Can you work these out from the model? Positions are in its coordinate system, mm. A direction names the side the tool comes from. Round coordinates to 2 decimals unless told otherwise and drop trailing zeros. Write each loop counter-clockwise with the first axis right and the second up, starting at its lowest first coordinate (ties: lowest second). Pieces come first, ordered by that corner, then holes. Notation, with made-up numbers: M 79,13 L 116,13 A28 cw 116,34 Z; hole C 8,-3 d2. An arc over 180 degrees is marked long. Use one line per item in the form item = value. Start each with the question number.
```python
from build123d import *

# Parameters (mm, degrees)
ESQUISSE1_W             = 37
ESQUISSE1_H             = 42.25
ESQUISSE1_R             = 6
BOSS_EXTRU_1_DEPTH      = 12
ESQUISSE2_R             = 6
ESQUISSE2_R_2           = 1.5
ENL_V_MAT_EXTRU_1_DEPTH = 3
ESQUISSE3_W             = 37
ESQUISSE3_H             = 12
ESQUISSE3_W_2           = 15.75
ESQUISSE3_R             = 2.75
BOSS_EXTRU_2_DEPTH      = 3
ESQUISSE4_W             = 37
ESQUISSE4_H             = 45.25
ESQUISSE4_R             = 8
ENL_V_MAT_EXTRU_2_DEPTH = 4
ESQUISSE4_3_R           = 8
ESQUISSE4_3_R_2         = 6
ESQUISSE4_3_R_3         = 1.5
ENL_V_MAT_EXTRU_4_DEPTH = 7
CONG_2_R                = 5
CONG_3_R                = 5
ESQUISSE5_R             = 2
ENL_V_MAT_EXTRU_5_DEPTH = 43.650652105
BOSS_EXTRU_3_START      = 2
ESQUISSE2_2_R           = 1.5
BOSS_EXTRU_3_DEPTH      = 2
SYM_TRIE1_OUTLINE_W     = 37
SYM_TRIE1_OUTLINE_H     = 45.25
SYM_TRIE1_OUTLINE_R     = 8
SYM_TRIE1_OUTLINE_R_2   = 2
SYM_TRIE1_OUTLINE_R_3   = 1.5
SYM_TRIE1_DEPTH         = 8
SYM_TRIE1_2_OUTLINE_W   = 15.75
SYM_TRIE1_2_OUTLINE_H   = 3
SYM_TRIE1_2_OUTLINE_R   = 8
SYM_TRIE1_2_OUTLINE_R_2 = 1.5
SYM_TRIE1_2_DEPTH       = 4.7499999
SYM_TRIE1_START         = 10.2500001
SYM_TRIE1_3_OUTLINE_W   = 15.75
SYM_TRIE1_3_OUTLINE_H   = 3
SYM_TRIE1_3_OUTLINE_R   = 1.5
SYM_TRIE1_3_DEPTH       = 1.7499999
SYM_TRIE1_START_2       = 1.13256
SYM_TRIE1_4_OUTLINE_R   = 8
SYM_TRIE1_4_OUTLINE_R_2 = 1.5
SYM_TRIE1_4_DEPTH       = 3.86744
SYM_TRIE1_START_3       = 8
SYM_TRIE1_5_OUTLINE_R   = 1.5
SYM_TRIE1_5_DEPTH       = 2.73256
SYM_TRIE1_START_4       = -24.125
SYM_TRIE1_6_DEPTH       = 3
ESQUISSE6_W             = 14
ESQUISSE6_H             = 45.25
ENL_V_MAT_EXTRU_6_DEPTH = 60.670580063


with BuildPart() as part:
    # Esquisse1 → Boss.-Extru.1 (new body)
    # profile 1 of 2: a face of its own
    with BuildSketch(Plane.XY):
        Rectangle(ESQUISSE1_W, ESQUISSE1_H)
        with Locations((3.4, 9.125)):
            Circle(ESQUISSE1_R, mode=Mode.SUBTRACT)
    # profile 2 of 2: a face of its own
    with BuildSketch(Plane.XY):
        with Locations((3.4, 9.125)):
            Circle(ESQUISSE1_R)
    extrude(amount=BOSS_EXTRU_1_DEPTH)

    # Esquisse2 → Enlèv. mat.-Extru.1 (cut)
    with BuildSketch(Plane.XY.offset(12)):
        with Locations((3.4, 9.125)):
            Circle(ESQUISSE2_R)
        with Locations((3.4, 9.125)):
            Circle(ESQUISSE2_R_2, mode=Mode.SUBTRACT)
    extrude(amount=-ENL_V_MAT_EXTRU_1_DEPTH, mode=Mode.SUBTRACT)

    # Esquisse3 → Boss.-Extru.2 (add)
    # profile 1 of 2: a face of its own
    with BuildSketch(Plane.XZ.offset(21.125)):
        with Locations((0, 6)):
            Rectangle(ESQUISSE3_W, ESQUISSE3_H)
    # profile 2 of 2: a face of its own
    with BuildSketch(Plane.XZ.offset(21.125)):
        with Locations((-26.375, 6)):
            Rectangle(ESQUISSE3_W_2, ESQUISSE3_H)
        with Locations((-29, 7.5)):
            Circle(ESQUISSE3_R, mode=Mode.SUBTRACT)
    extrude(amount=BOSS_EXTRU_2_DEPTH)

    # Esquisse4 → Enlèv. mat.-Extru.2 (cut)
    with BuildSketch(Plane.XY.offset(12)):
        with Locations((0, -1.5)):
            Rectangle(ESQUISSE4_W, ESQUISSE4_H)
        with Locations((3.4, 9.125)):
            Circle(ESQUISSE4_R, mode=Mode.SUBTRACT)
    extrude(amount=-ENL_V_MAT_EXTRU_2_DEPTH, mode=Mode.SUBTRACT)

    # Esquisse4<3> → Enlèv. mat.-Extru.4 (cut)
    # profile 1 of 2: a face of its own
    with BuildSketch(Plane.XY.offset(12)):
        with Locations((3.4, 9.125)):
            Circle(ESQUISSE4_3_R)
        with Locations((3.4, 9.125)):
            Circle(ESQUISSE4_3_R_2, mode=Mode.SUBTRACT)
    # profile 2 of 2: a face of its own
    with BuildSketch(Plane.XY.offset(12)):
        with Locations((3.4, 9.125)):
            Circle(ESQUISSE4_3_R_2)
        with Locations((3.4, 9.125)):
            Circle(ESQUISSE4_3_R_3, mode=Mode.SUBTRACT)
    extrude(amount=-ENL_V_MAT_EXTRU_4_DEPTH, mode=Mode.SUBTRACT)

    # Congé2
    # the kernel refuses this fillet: 5 mm, written as the material it adds along each edge
    with BuildSketch(Plane(origin=(-18.5, -24.125, 8), x_dir=(1.5667467323505199e-12, 0, 1.0), z_dir=(0, 1, 0))) as cong_2_piece_1:
        with BuildLine():
            CenterArc((5, 4.898979486), CONG_2_R, 180, 78.463040967)
            Line((0, 4.898979486), (0, 0))
            Line((0, 0), (4, 0))
        make_face()
    extrude(amount=3)

    # Congé3
    cong_3_edges = [part.edges().sort_by_distance(p)[0] for p in [
        (-18.5, -22.625, 12),
    ]]
    fillet(cong_3_edges, radius=CONG_3_R)

    # Esquisse5 → Enlèv. mat.-Extru.5 (cut, through all)
    with BuildSketch(Plane.XY.offset(8)):
        with Locations((-12, 16.625)):
            Circle(ESQUISSE5_R)
        with Locations((-12, 4.625)):
            Circle(ESQUISSE5_R)
        with Locations((15.5, 10.625)):
            Circle(ESQUISSE5_R)
    extrude(amount=-ENL_V_MAT_EXTRU_5_DEPTH, mode=Mode.SUBTRACT)

    # Esquisse2<2> → Boss.-Extru.3 (add)
    with BuildSketch(Plane.XY.offset(12).offset(BOSS_EXTRU_3_START)):
        with Locations((3.4, 9.125)):
            Circle(ESQUISSE2_2_R)
    extrude(amount=-BOSS_EXTRU_3_DEPTH)

    # Symétrie1: read off the stored shape, not the designer's step
    # Symétrie1 outline → Symétrie1 (add)
    # profile 1 of 2: a face of its own
    with BuildSketch(Plane.XY):
        with Locations((37, -1.5)):
            Rectangle(SYM_TRIE1_OUTLINE_W, SYM_TRIE1_OUTLINE_H)
        with Locations((33.6, 9.125)):
            Circle(SYM_TRIE1_OUTLINE_R, mode=Mode.SUBTRACT)
        with Locations((21.5, 10.625)):
            Circle(SYM_TRIE1_OUTLINE_R_2, mode=Mode.SUBTRACT)
        with Locations((49, 4.625)):
            Circle(SYM_TRIE1_OUTLINE_R_2, mode=Mode.SUBTRACT)
        with Locations((49, 16.625)):
            Circle(SYM_TRIE1_OUTLINE_R_2, mode=Mode.SUBTRACT)
    # profile 2 of 2: a face of its own
    with BuildSketch(Plane.XY):
        with Locations((33.6, 9.125)):
            Circle(SYM_TRIE1_OUTLINE_R_3)
    extrude(amount=SYM_TRIE1_DEPTH)

    # Sym_trie1 2 outline → Sym_trie1 2 (add)
    # profile 1 of 2: a face of its own
    with BuildSketch(Plane.XY):
        with Locations((63.375, -22.625)):
            Rectangle(SYM_TRIE1_2_OUTLINE_W, SYM_TRIE1_2_OUTLINE_H)
    # profile 2 of 2: a face of its own
    with BuildSketch(Plane.XY):
        with Locations((33.6, 9.125)):
            Circle(SYM_TRIE1_2_OUTLINE_R)
        with Locations((33.6, 9.125)):
            Circle(SYM_TRIE1_2_OUTLINE_R_2, mode=Mode.SUBTRACT)
    extrude(amount=SYM_TRIE1_2_DEPTH)

    # Sym_trie1 4 outline → Sym_trie1 4 (add)
    with BuildSketch(Plane.XY.offset(SYM_TRIE1_START_2)):
        with Locations((33.6, 9.125)):
            Circle(SYM_TRIE1_4_OUTLINE_R)
        with Locations((33.6, 9.125)):
            Circle(SYM_TRIE1_4_OUTLINE_R_2, mode=Mode.SUBTRACT)
    extrude(amount=SYM_TRIE1_4_DEPTH)



with BuildPart() as body_2:
    # Sym_trie1 3 outline → Sym_trie1 3 (new body)
    with BuildSketch(Plane.XY.offset(SYM_TRIE1_START)):
        with Locations((63.375, -22.625)):
            Rectangle(SYM_TRIE1_3_OUTLINE_W, SYM_TRIE1_3_OUTLINE_H)
        with Locations((33.6, 9.125)):
            Circle(SYM_TRIE1_3_OUTLINE_R)
    extrude(amount=SYM_TRIE1_3_DEPTH)


with BuildPart() as part_1:
    add(part.part)

    add(body_2.part)  # Sym_trie1 5 merges body 2
    # Sym_trie1 5 outline → Sym_trie1 5 (add)
    with BuildSketch(Plane.XY.offset(SYM_TRIE1_START_3)):
        with Locations((33.6, 9.125)):
            Circle(SYM_TRIE1_5_OUTLINE_R)
    extrude(amount=SYM_TRIE1_5_DEPTH)

    # Sym_trie1 6 outline → Sym_trie1 6 (add)
    with BuildSketch(Plane(origin=(0, 0, 0), x_dir=(1, 0, 0), z_dir=(0, 1, 0)).offset(SYM_TRIE1_START_4)):
        with BuildLine():
            Line((66, -10.25), (71.25, -10.2500001))
            Line((71.25, -10.2500001), (71.25, -4.7499999))
            Line((71.25, -4.7499999), (66, -4.75))
            ThreePointArc((66, -4.75), (68.75, -7.5), (66, -10.25))
        make_face()
        with BuildLine():
            Line((55.5, -10.2500001), (66, -10.25))
            ThreePointArc((66, -10.25), (63.25, -7.5), (66, -4.75))
            Line((66, -4.75), (55.5, -4.7499999))
            Line((55.5, -4.7499999), (55.5, -10.2500001))
        make_face()
    extrude(amount=SYM_TRIE1_6_DEPTH)

    # Esquisse6 → Enlèv. mat.-Extru.6 (cut, through all)
    with BuildSketch(Plane(origin=(18.5, 0, 0), x_dir=(0, 0, -1), z_dir=(1, 0, 0))):
        with Locations((-7, -1.5)):
            Rectangle(ESQUISSE6_W, ESQUISSE6_H)
    extrude(amount=-ENL_V_MAT_EXTRU_6_DEPTH, mode=Mode.SUBTRACT)


solid = part_1.part
```
1. Please list where these lines run through material, in increasing order: line 1 along Y through (x, z) = (49, 4.5) (3 decimals); line 2 along Y through (x, z) = (21.5, 5.25) (3 decimals); line 3 along X through (y, z) = (-22.35, 7.5).
2. Which directions (+Z, -Z, +X, -X, +Y, -Y) give clear straight access to the entire face, cutting with the end or side of a thin tool? Please do faces 5 (the face through (32.41, 8.21, 8.45)), 6 (the face through (63, -21.125, 6)), 7 (the face through (45, -24.125, 5)).
3. If we section it at D-D (x = 33.6): List the corners of the cut face in (y, z) for me (3 decimals).
4. If we section it at A-A (x = 21.5): List the corners of the cut face in (y, z) for me (3 decimals), and give its area (3 significant figures).
5. If we section it at C-C (z = 11): List the corners of the cut face in (x, y) for me (3 decimals).
6. If we section it at B-B (x = 49): List the corners of the cut face in (y, z) for me (3 decimals).
7. Will these pins go through, and if not, where does the flat tip stop? pin 1 (5 mm diameter, centred on x = 49, y = 4.625, fed in from +Z); pin 2 (4 mm diameter, centred on y = 10, z = 4, fed in from +X); pin 3 (6 mm diameter, centred on x = 67, z = 8.5, fed in from +Y) (3 decimals).
8. If we mould it in two halves opening along Y, with no side actions, what happens to faces 1 (the face through (27.25, 4.26, 6.48)), 2 (the face through (55.5, -23, 10)), 3 (the face through (21.24, 12.61, 3.94)), 4 (the face through (37, 21.125, 4))? For each: pulls with the +Y half, pulls with the -Y half, needs draft (parallel to the pull), parting line crosses it, or undercut.
Model answer:
q1.line_1 = -24.125 to 2.625, 6.625 to 14.625, 18.625 to 21.125
q1.line_2 = -24.125 to 8.625, 12.625 to 21.125
q1.line_3 = 18.5 to 63.25, 68.75 to 71.25
q2.face_5 = +Z
q2.face_6 = +Z, -Z, +X, +Y
q2.face_7 = +Z, -Z, +X, -X, -Y
q3.outline = M -24.125,0 L 21.125,0 L 21.125,8 L 17.125,8 L 17.125,5 L 10.625,5 L 10.625,12 L 7.625,12 L 7.625,5 L 1.125,5 L 1.125,8 L -24.125,8 Z
q4.outline = M -24.125,0 L 8.625,0 L 8.625,8 L -24.125,8 Z; M 12.625,0 L 21.125,0 L 21.125,8 L 12.625,8 Z
q4.area = 330 mm2
q5.outline = C 33.6,9.125 d3; M 55.5,-24.125 L 71.25,-24.125 L 71.25,-21.125 L 55.5,-21.125 Z
q6.outline = M -24.125,0 L 2.625,0 L 2.625,8 L -24.125,8 Z; M 6.625,0 L 14.625,0 L 14.625,8 L 6.625,8 Z; M 18.625,0 L 21.125,0 L 21.125,8 L 18.625,8 Z
q7.pin_1 = 8
q7.pin_2 = 55.5
q7.pin_3 = -21.125
q8.face_1 = undercut
q8.face_2 = needs draft
q8.face_3 = undercut
q8.face_4 = pulls with the +Y half
